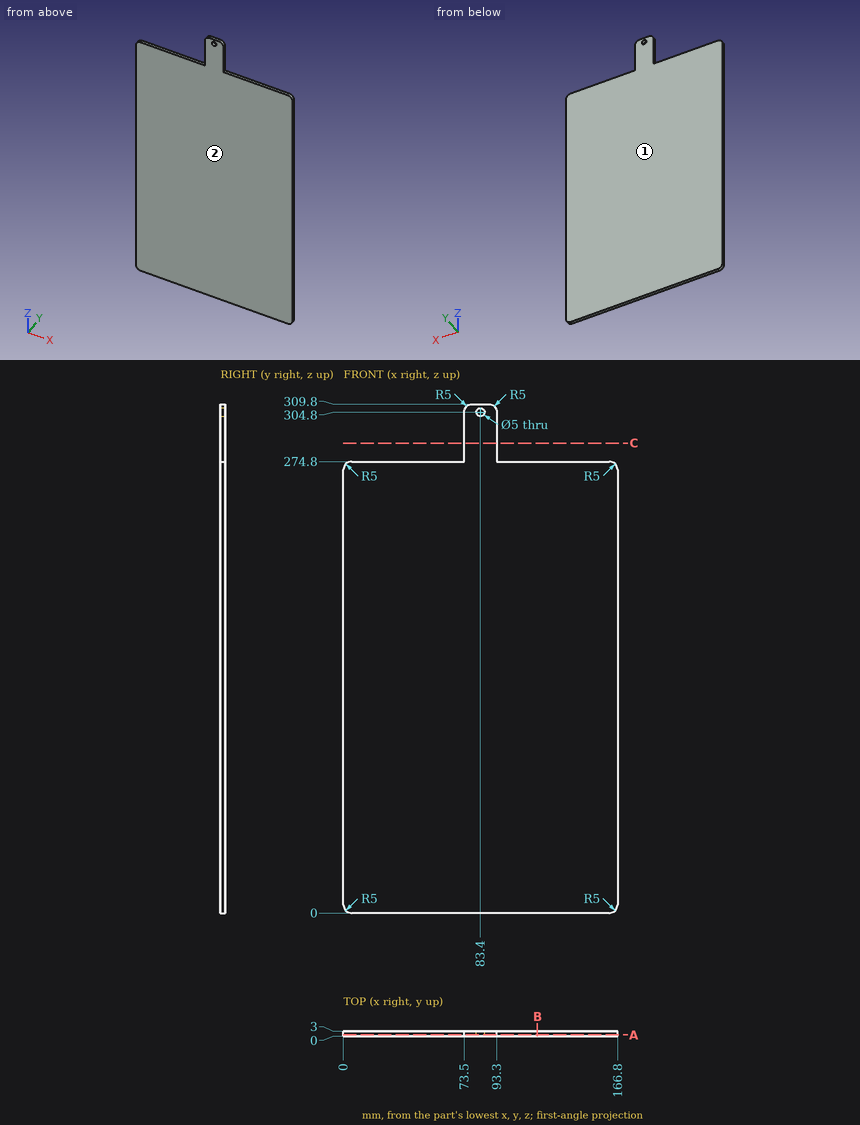
Job drawing, mm, ordinate dimensions from the low corner. One solid piece. Coordinates: 2 decimals unless noted, no trailing zeros. Loops run counter-clockwise (first coordinate to the right, second up) from the corner with the lowest first, then second, coordinate; pieces in that order, holes last. Notation, with made-up numbers: (-35, 83.25) -> (21, 83.25) arc R21 ccw to (21, 120.25) -> close; hole circle Ø4 at (60.5, 77.25). An arc over 180 degrees is marked (long way). One line per item, written item: value.
1. Slice it at A-A on y = 0.7. Write the cut outline in (x, z).
Answers:
outline: (0, 5) arc R5 ccw to (5, 0) -> (161.8, 0) arc R5 ccw to (166.8, 5) -> (166.8, 269.8) arc R5 ccw to (161.8, 274.8) -> (93.3, 274.8) -> (93.3, 304.8) arc R5 ccw to (88.3, 309.8) -> (78.5, 309.8) arc R5 ccw to (73.5, 304.8) -> (73.5, 274.8) -> (5, 274.8) arc R5 ccw to (0, 269.8) -> close; hole circle Ø5 at (83.4, 304.8)
2. Slice it at B-B on x = 118. Write the cut outline in (y, z).
Answers:
outline: (0, 0) -> (3, 0) -> (3, 274.8) -> (0, 274.8) -> close
3. Slice it at C-C on z = 286. Write the cut outline in (x, y), and give its area (3 significant figures).
Answers:
outline: (73.5, 0) -> (93.3, 0) -> (93.3, 3) -> (73.5, 3) -> close
area: 59.4 mm^2
4. Pull direction Y, two halves, no side cores. Call the marked faces 1 and 2: pulls with the +Y half, pulls with the -Y half, needs draft (parallel to the pull), parting line crosses it, or undercut.
Answers:
face 1: pulls with the +Y half
face 2: pulls with the -Y half
5. Flat gauge pins, fed straight in: P1, Ø6, axis at x = 79, z = 112.5, coming from the -Y side; P2, Ø0.9, axis at x = 42.5, y = 2, coming from the +Z side. Where does each tip first touch, or does it go through?
Answers:
P1: stops at y = 0
P2: stops at z = 274.8
6. Drill centre lines: line 1 (X direction, y = 1.85, z = 304.8); line 2 (Z direction, x = 83.4, y = 1); line 3 (Z direction, x = 38.5, y = 2.6). Where is each one in solid material? Low to high. Write a range as [from, to].
Answers:
line 1: x = [73.5, 80.9], [85.9, 93.3]
line 2: z = [0, 302.3], [307.3, 309.8]
line 3: z = [0, 274.8]
